Verification items for the finished model (mm, model axes). Face numbers are marked on the shaded views. A direction names the side the tool comes from. Round coordinates to 2 decimals unless told otherwise and drop trailing zeros. Order: outer loops, then holes, each group sorted by start corner. A loop starts at its lowest first (then second) coordinate and runs counter-clockwise, first axis right, second up. Notation, with made-up numbers: (6.25, 29) -> (37.25, 29) arc R17 ccw to (37.25, 40) -> close; hole circle Ø10 at (56.5, 79). An arc over 180 degrees is marked (long way). Return JSON: item names as keys, results as strings. Group by question number.
1) Tool access check on the marked faces 1, 2 and 3. Record the directions out of +Z, -Z, +X, -X, +Y, -Y that give a thin tool (end or side, any length) a straight path to the whole face; none if there is none.
2) Scan lines: L1, parallel to Y at x = -4.5, z = 4.25; L2, parallel to X at y = -3, z = -5.25; L3, parallel to X at y = 1, z = 4.25. Record each from-to range of solid material in increasing order.
3) Section check B-B on z = 0. Enter the section's corners in (x, y).
4) Depth check by flat-ended pin: pin 1 (5 mm diameter, centred on y = 5, z = 5.5, fed in from +X); pin 2 (6 mm diameter, centred on x = 6, y = -4, fed in from -Z); pin 3 (1 mm diameter, centred on x = 3.5, z = 2.5, fed in from -Y); pin 4 (5 mm diameter, centred on x = 2, z = -3, fed in from -Y). Enter the tip coordinate at first touch or a pass-through.
5) Section check A-A on y = 3.25. Enter the section's corners in (x, z), plus the area to 3 significant figures.
6) Draft check along X on the marked faces 4, 5, 6 and 7. Enter one of: pulls with the +X half, pulls with the -X half, needs draft (parallel to the pull), parting line crosses it, or undercut.
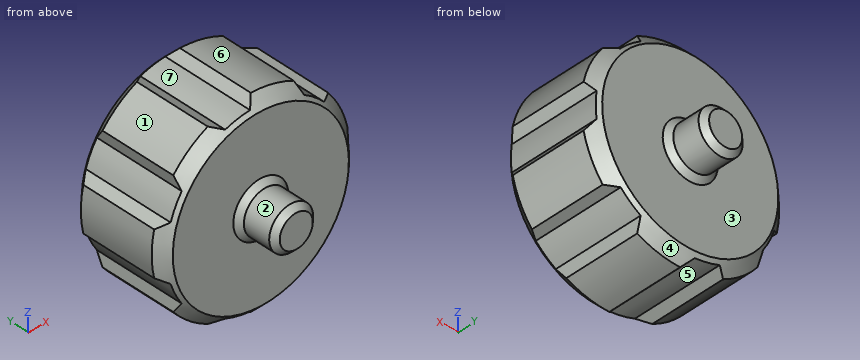
```python
from build123d import *

# Parameters (mm, degrees)
CORTAR_EXTRUIR1_DEPTH      = 18.839562775
CORTAR_EXTRUIR1_DEPTH_BACK = 18.839562775


with BuildPart() as part:
    # Croquis1 → Revolución1 (revolve)
    with BuildSketch(Plane.XY, mode=Mode.PRIVATE) as revoluci_n1_sk:
        Polygon((0, -8), (0, 8), (-1.5, 8), (-2, 7.5), (-2, 5), (-2.5, 4.5), (-8, 4.5), (-9, 3.5), (-9, -3.5), (-8, -4.5), (-2.5, -4.5), (-2, -5), (-2, -7.5), (-1.5, -8), align=None)
    revolve(revoluci_n1_sk.sketch.rotate(Axis((0, -8, 0), (0, 1, 0)), 270), axis=Axis((0, -8, 0), (0, 1, 0)))

    # Croquis2 → Cortar-Extruir1 (cut, two sides: drawn at the far end of the back side and taken through both)
    with BuildSketch(Plane(origin=(0, 4.5, 0), x_dir=(1, 0, 0), z_dir=(0, 1, 0)).offset(-CORTAR_EXTRUIR1_DEPTH_BACK)):
        with BuildLine():
            Line((0, 9), (-0.7, 8.278295995))
            ThreePointArc((-0.7, 8.278295995), (-1.848968457, 8.099475306), (-2.961715623, 7.761985903))
            Line((-2.961715623, 7.761985903), (-3.904953652, 8.108719811))
            ThreePointArc((-3.904953652, 8.108719811), (-2.002688406, 8.77435121), (0, 9))
        make_face()
        with BuildLine():
            Line((3.904953652, 8.108719811), (4.221965458, 7.155081569))
            ThreePointArc((4.221965458, 7.155081569), (5.179611809, 6.495522003), (6.035789569, 5.708715168))
            Line((6.035789569, 5.708715168), (7.036483342, 5.611408217))
            ThreePointArc((7.036483342, 5.611408217), (5.611408217, 7.036483342), (3.904953652, 8.108719811))
        make_face()
        with BuildLine():
            Line((8.77435121, 2.002688406), (8.226420437, 1.160254876))
            ThreePointArc((8.226420437, 1.160254876), (8.307838738, 0.000308148), (8.226506485, -1.159644618))
            Line((8.226506485, -1.159644618), (8.77435121, -2.002688406))
            ThreePointArc((8.77435121, -2.002688406), (9, 0), (8.77435121, 2.002688406))
        make_face()
        with BuildLine():
            Line((7.036483342, -5.611408217), (6.036213038, -5.708267403))
            ThreePointArc((6.036213038, -5.708267403), (5.180093648, -6.495137749), (4.222496227, -7.154768354))
            Line((4.222496227, -7.154768354), (3.904953652, -8.108719811))
            ThreePointArc((3.904953652, -8.108719811), (5.611408217, -7.036483342), (7.036483342, -5.611408217))
        make_face()
        with BuildLine():
            Line((0, -9), (-0.699385895, -8.2783479))
            ThreePointArc((-0.699385895, -8.2783479), (-1.848367613, -8.099612444), (-2.961139812, -7.762205588))
            Line((-2.961139812, -7.762205588), (-3.904953652, -8.108719811))
            ThreePointArc((-3.904953652, -8.108719811), (-2.002688406, -8.77435121), (0, -9))
        make_face()
        with BuildLine():
            Line((-7.036483342, -5.611408217), (-6.908332984, -4.614663581))
            ThreePointArc((-6.908332984, -4.614663581), (-7.484970362, -3.604913767), (-7.914977177, -2.524543695))
            Line((-7.914977177, -2.524543695), (-8.77435121, -2.002688406))
            ThreePointArc((-8.77435121, -2.002688406), (-8.108719811, -3.904953652), (-7.036483342, -5.611408217))
        make_face()
        with BuildLine():
            Line((-8.77435121, 2.002688406), (-7.915164432, 2.523956536))
            ThreePointArc((-7.915164432, 2.523956536), (-7.485237762, 3.604358504), (-6.908675292, 4.614151092))
            Line((-6.908675292, 4.614151092), (-7.036483342, 5.611408217))
            ThreePointArc((-7.036483342, 5.611408217), (-8.108719811, 3.904953652), (-8.77435121, 2.002688406))
        make_face()
    extrude(amount=CORTAR_EXTRUIR1_DEPTH + CORTAR_EXTRUIR1_DEPTH_BACK, mode=Mode.SUBTRACT)


solid = part.part
```
Check result:
{
 "1": {"face 1": "+Z, -X, +Y, -Y", "face 2": "-Y", "face 3": "+Y"},
 "2": {"L1": "-4.5 to 4.5", "L2": "-6.99 to 7.31", "L3": "-7.14 to 7.93"},
 "3": {"outline": "(-9, -3.5) -> (-8, -4.5) -> (-2.5, -4.5) -> (-2, -5) -> (-2, -7.5) -> (-1.5, -8) -> (1.5, -8) -> (2, -7.5) -> (2, -5) -> (2.5, -4.5) -> (8, -4.5) -> (8.31, -4.19) -> (8.31, 4.19) -> (8, 4.5) -> (2.5, 4.5) -> (2, 5) -> (2, 7.5) -> (1.5, 8) -> (-1.5, 8) -> (-2, 7.5) -> (-2, 5) -> (-2.5, 4.5) -> (-8, 4.5) -> (-9, 3.5) -> close"},
 "4": {"pin 1": "x = 8.29", "pin 2": "z = -8.47", "pin 3": "y = -4.5", "pin 4": "y = -8"},
 "5": {"outline": "(-8.77, -2) -> (-7.92, -2.52) arc R8.31 ccw to (-6.91, -4.61) -> (-7.04, -5.61) arc R9 ccw to (-3.9, -8.11) -> (-2.96, -7.76) arc R8.31 ccw to (-0.7, -8.28) -> (0, -9) arc R9 ccw to (3.9, -8.11) -> (4.22, -7.16) arc R8.31 ccw to (6.04, -5.71) -> (7.04, -5.61) arc R9 ccw to (8.77, -2) -> (8.23, -1.16) arc R8.31 ccw to (8.23, 1.16) -> (8.77, 2) arc R9 ccw to (7.04, 5.61) -> (6.04, 5.71) arc R8.31 ccw to (4.22, 7.15) -> (3.9, 8.11) arc R9 ccw to (0, 9) -> (-0.7, 8.28) arc R8.31 ccw to (-2.96, 7.76) -> (-3.9, 8.11) arc R9 ccw to (-7.04, 5.61) -> (-6.91, 4.61) arc R8.31 ccw to (-7.91, 2.52) -> (-8.77, 2) arc R9 ccw to start", "area": "239 mm^2"},
 "6": {"face 4": "parting line crosses it", "face 5": "undercut", "face 6": "pulls with the +X half", "face 7": "undercut"}
}
